Could you check a few things on this model? Use its own coordinates, in mm. A direction names the side the tool comes from. Give positions to 0.01 mm unless a question says otherwise; leave off trailing zeros. Write each loop counter-clockwise with the first axis right and the second up, starting at its lowest first coordinate (ties: lowest second). Pieces come first, ordered by that corner, then holes. Notation, with made-up numbers: (51.5, -20.5) - (106.5, -20.5) arc R6 cw to (106.5, -14.5) - close; hole circle Ø11 at (-9, -40). An arc over 180 degrees is marked (long way). Answer in a Markdown table with one row per item.
from build123d import *

# Parameters (mm, degrees)
BASE_EXTRUDE_DEPTH             = 12.7
F_9_16_0_5625_DIAMETER_HOLE1_D = 14.2875
CUT_EXTRUDE1_REACH             = 14.7
BOSS_EXTRUDE1_DEPTH            = 25.4
F_1_2_20_TAPPED_HOLE1_D        = 12.7
CUT_EXTRUDE2_DEPTH             = 39.1
CUT_EXTRUDE3_DEPTH             = 39.1
F_1_2_20_TAPPED_HOLE2_D        = 12.7
CUT_EXTRUDE4_DEPTH             = 25.4


with BuildPart() as part:
    # Sketch1 → Base-Extrude (new body)
    with BuildSketch(Plane.XY):
        Polygon((58.12164787, 111.098459585), (-37.201684746, 66.648459585), (-37.201684746, -66.701540415), (264.657388756, -66.701540415), (264.657388756, 66.648459585), (169.334056139, 111.098459585), align=None)
    extrude(amount=BASE_EXTRUDE_DEPTH)

    # 9/16 (0.5625) Diameter Hole1 (through all)
    with Locations(Plane.XY.offset(12.7)):
        with Locations((251.957388756, -9.551540415), (251.957388756, 41.248459585)):
            f_9_16_0_5625_diameter_hole1 = Hole(F_9_16_0_5625_DIAMETER_HOLE1_D / 2)

    # Sketch8 → Cut-Extrude1 (cut, up to next)
    with BuildSketch(Plane.XY.offset(12.7), mode=Mode.PRIVATE) as cut_extrude1_sk1:
        with BuildLine():
            Line((5.818295254, -25.4), (5.818295254, -66.701540415))
            Line((5.818295254, -66.701540415), (221.718295254, -66.701540415))
            Line((221.718295254, -66.701540415), (221.718295254, -25.4))
            ThreePointArc((221.718295254, -25.4), (214.278807496, -7.439487758), (196.318295254, 0))
            Line((196.318295254, 0), (150.956476278, 0))
            Line((150.956476278, 0), (138.302811241, 47.224120819))
            ThreePointArc((138.302811241, 47.224120819), (113.768295254, 66.050117074), (89.233779266, 47.224120819))
            Line((89.233779266, 47.224120819), (76.580114229, 0))
            Line((76.580114229, 0), (31.218295254, 0))
            ThreePointArc((31.218295254, 0), (13.257783011, -7.439487758), (5.818295254, -25.4))
        make_face()
    cut_extrude1_tool1 = extrude(cut_extrude1_sk1.sketch, amount=-CUT_EXTRUDE1_REACH, mode=Mode.PRIVATE) & part.part
    add(cut_extrude1_tool1.solids().sort_by_distance((113.768295, -21.271265, 12.7))[0], mode=Mode.SUBTRACT)

    # Mirror3: 9/16 (0.5625) Diameter Hole1 across plane
    add(f_9_16_0_5625_diameter_hole1.mirror(Plane(origin=(113.768295254, 0, 0), x_dir=(0, 0, 1), z_dir=(1, 0, 0))), mode=Mode.SUBTRACT)

    # Sketch10 → Boss-Extrude1 (add)
    with BuildSketch(Plane(origin=(0, 0, 0), x_dir=(-1, 0, 0), z_dir=(0, 0, -1))):
        Polygon((-169.334056139, 111.098459585), (-58.12164787, 111.098459585), (33.824515248, 68.223259585), (-261.280219258, 68.223259585), align=None)
    extrude(amount=BOSS_EXTRUDE1_DEPTH)

    # 1/2-20 Tapped Hole1 (through all)
    with Locations(Plane(origin=(0, 111.098459585, 0), x_dir=(-1, 0, 0), z_dir=(0, 1, 0))):
        with Locations((-113.69684787, -12.7)):
            Hole(F_1_2_20_TAPPED_HOLE1_D / 2)

    # Sketch13 → Cut-Extrude2 (cut, through all)
    with BuildSketch(Plane.XY.offset(12.7)):
        with BuildLine():
            Line((250.369888756, -2.407790415), (253.544888756, -2.407790415))
            ThreePointArc((253.544888756, -2.407790415), (260.688638756, -9.551540415), (253.544888756, -16.695290415))
            Line((253.544888756, -16.695290415), (250.369888756, -16.695290415))
            ThreePointArc((250.369888756, -16.695290415), (243.226138756, -9.551540415), (250.369888756, -2.407790415))
        make_face()
    cut_extrude2 = extrude(amount=-CUT_EXTRUDE2_DEPTH, mode=Mode.SUBTRACT)

    # Sketch14 → Cut-Extrude3 (cut, through all)
    with BuildSketch(Plane.XY.offset(12.7)):
        with BuildLine():
            Line((253.532188756, 48.392209585), (250.382588756, 48.392209585))
            ThreePointArc((250.382588756, 48.392209585), (243.238838756, 41.248459585), (250.382588756, 34.104709585))
            Line((250.382588756, 34.104709585), (253.532188756, 34.104709585))
            ThreePointArc((253.532188756, 34.104709585), (260.675938756, 41.248459585), (253.532188756, 48.392209585))
        make_face()
    cut_extrude3 = extrude(amount=-CUT_EXTRUDE3_DEPTH, mode=Mode.SUBTRACT)

    # Mirror4: Cut-Extrude2, Cut-Extrude3 across plane
    add(cut_extrude2.mirror(Plane(origin=(113.768295254, 0, 0), x_dir=(0, 0, 1), z_dir=(1, 0, 0))), mode=Mode.SUBTRACT)
    add(cut_extrude3.mirror(Plane(origin=(113.768295254, 0, 0), x_dir=(0, 0, 1), z_dir=(1, 0, 0))), mode=Mode.SUBTRACT)

    # 1/2-20 Tapped Hole2 (through all)
    with Locations(Plane.XY.offset(12.7)):
        with Locations((38.998315254, 41.248459585), (188.457388756, 41.248459585)):
            Hole(F_1_2_20_TAPPED_HOLE2_D / 2)

    # Sketch17 → Cut-Extrude4 (cut)
    with BuildSketch(Plane(origin=(0, 0, -25.4), x_dir=(-1, 0, 0), z_dir=(0, 0, -1))):
        with BuildLine():
            Line((-132.777852005, 68.223259585), (-94.677852005, 68.223259585))
            Line((-94.677852005, 68.223259585), (-94.677852005, 87.273259585))
            ThreePointArc((-94.677852005, 87.273259585), (-97.467659914, 94.008451676), (-104.202852005, 96.798259585))
            Line((-104.202852005, 96.798259585), (-123.252852005, 96.798259585))
            ThreePointArc((-123.252852005, 96.798259585), (-129.988044096, 94.008451676), (-132.777852005, 87.273259585))
            Line((-132.777852005, 87.273259585), (-132.777852005, 68.223259585))
        make_face()
    extrude(amount=-CUT_EXTRUDE4_DEPTH, mode=Mode.SUBTRACT)


solid = part.part
1) We'd pull the mould along Y, two halves only. Please class faces 1 (the face through (119.563, 103.848, -15.132)), 2 (the face through (243.228, -9.709, 6.439)), 3 (the face through (-15.69, -9.71, 6.44)), 4 (the face through (30, 68.223, -13)): +Y half, -Y half, draft (parallel to the pull), parting line (faces both ways), or undercut.
Check values:
| item | result |
|---|---|
| face 1 | draft |
| face 2 | undercut |
| face 3 | undercut |
| face 4 | -Y half |
2) Imagine slicing it at C-C (x = 217). List the corners of the cut face in (y, z) for me.
Check values:
| item | result |
|---|---|
| outline | (-10.65, 0) - (68.22, 0) - (68.22, -25.4) - (88.87, -25.4) - (88.87, 12.7) - (-10.65, 12.7) - close |
3) If I drill on line 1 (X direction, y = -32, z = 8); line 2 (Z direction, x = 249.5, y = -54.5); line 3 (Y direction, x = 144, z = -6), over which ranges is the centre line in solid material (lowest first)?
Check values:
| item | result |
|---|---|
| line 1 | x = -37.2 to 5.82, 221.72 to 264.66 |
| line 2 | z = 0 to 12.7 |
| line 3 | y = 68.22 to 111.1 |
4) Imagine slicing it at D-D (x = 179). List the corners of the cut face in (y, z) for me, then the cut area to 3 significant figures.
Check values:
| item | result |
|---|---|
| outline | (0, 0) - (68.22, 0) - (68.22, -25.4) - (106.59, -25.4) - (106.59, 12.7) - (0, 12.7) - close |
| area | 2,330 mm2 |
5) Imagine slicing it at A-A (z = -12.7). List the corners of the cut face in (x, y) for me (3 decimals).
Check values:
| item | result |
|---|---|
| outline | (-33.825, 68.223) - (94.678, 68.223) - (94.678, 87.273) arc R9.525 cw to (104.203, 96.798) - (107.347, 96.798) - (107.347, 111.098) - (58.122, 111.098) - close; (120.047, 96.798) - (123.253, 96.798) arc R9.525 cw to (132.778, 87.273) - (132.778, 68.223) - (261.28, 68.223) - (169.334, 111.098) - (120.047, 111.098) - close |
6) On a 3-axis mill with a long thin cutter (end or side, diameter ignored), from which of +Z, -Z, +X, -X, +Y, -Y can I reach the whole of each face in a straight line? I mean faces 5 (the face through (107, 96.798, -13)), 6 (the face through (214.475, -7.638, 6.439)), 7 (the face through (196, 68.223, -13)), 8 (the face through (112, 99, -25.4)), 9 (the face through (260.674, 41.091, 6.439)). Say none if no direction works.
Check values:
| item | result |
|---|---|
| face 5 | -Z, -Y |
| face 6 | +Z, -Z, -Y |
| face 7 | -Z, +X, -X, -Y |
| face 8 | -Z, +X, -X, +Y, -Y |
| face 9 | +Z, -Z |
7) Will these pins go through, and if not, where does the flat tip stop? P1, Ø7.5, axis at x = 226.5, z = -19, coming from the -Y side; P2, Ø11.5, axis at x = 188.46, y = 41.25, coming from the +Z side; P3, Ø2.5, axis at x = 251.5, z = 6.5, coming from the +Y side; P4, Ø15, axis at y = 78, z = -10, coming from the +X side.
Check values:
| item | result |
|---|---|
| P1 | stops at y = 68.22 |
| P2 | passes through |
| P3 | stops at y = 73.37 |
| P4 | stops at x = 256.4 |
8) Imagine slicing it at B-B (y = 21.5). List the corners of the cut face in (x, z) for me, then the cut area to 3 significant figures.
Check values:
| item | result |
|---|---|
| outline | (-37.2, 0) - (82.34, 0) - (82.34, 12.7) - (-37.2, 12.7) - close; (145.2, 0) - (264.66, 0) - (264.66, 12.7) - (145.2, 12.7) - close |
| area | 3,040 mm2 |
